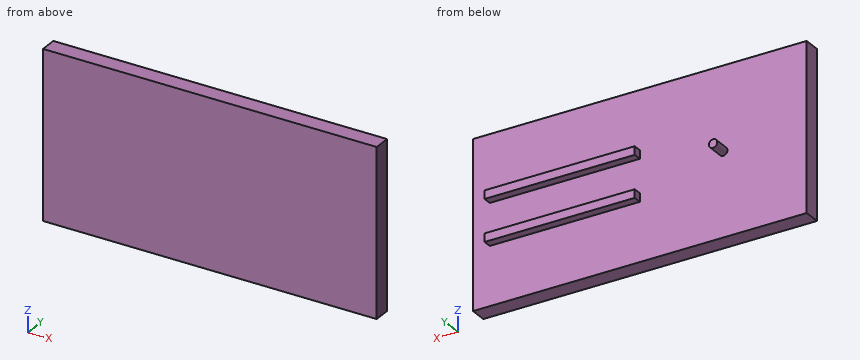
```python
from build123d import *

# Parameters (mm, degrees)
SKETCH1_W           = 200
SKETCH1_H           = 100
BOSS_EXTRUDE1_DEPTH = 10
SKETCH2_W           = 90
SKETCH2_H           = 5
BOSS_EXTRUDE2_DEPTH = 5
SKETCH2_3_R         = 2.5
BOSS_EXTRUDE3_DEPTH = 10


with BuildPart() as part:
    # Sketch1 → Boss-Extrude1 (new body)
    with BuildSketch(Plane(origin=(0, 0, 0), x_dir=(1, 0, 0), z_dir=(0, 1, 0))):
        Rectangle(SKETCH1_W, SKETCH1_H)
    extrude(amount=BOSS_EXTRUDE1_DEPTH)

    # Sketch2 → Boss-Extrude2 (add)
    with BuildSketch(Plane(origin=(0, 10, 0), x_dir=(1, 0, 0), z_dir=(0, 1, 0))):
        with Locations((45, 12.5)):
            Rectangle(SKETCH2_W, SKETCH2_H)
        with Locations((45, -12.5)):
            Rectangle(SKETCH2_W, SKETCH2_H)
    extrude(amount=BOSS_EXTRUDE2_DEPTH)

    # Sketch2_3 → Boss-Extrude3 (add)
    with BuildSketch(Plane(origin=(0, 10, 0), x_dir=(1, 0, 0), z_dir=(0, 1, 0))):
        with Locations(Location((-50, 0, 0), (0, 0, 90))):
            Circle(SKETCH2_3_R)
    extrude(amount=BOSS_EXTRUDE3_DEPTH)


solid = part.part
```
Build history of the part. All positions in model axes, mm. Round coordinates to 2 decimals unless told otherwise and drop trailing zeros. Order: outer loops, then holes, each group sorted by start corner. A loop starts at its lowest first (then second) coordinate and runs counter-clockwise, first axis right, second up. Notation, with made-up numbers: (21, 35.25) - (31, 35.25) arc R34 ccw to (31, 72.25) - close; hole circle Ø8 at (65.25, 1.5). An arc over 180 degrees is marked (long way). Use a Markdown table: item, result.
1) Flat gauge pins, fed straight in: pin 1 Ø1.5 at (x, y) = (36, 12) entering from -Z; pin 2 Ø10 at (x, z) = (-68, 10) entering from +Y; pin 3 Ø1.5 at (x, z) = (63.5, -12) entering from +Y. Where does each tip first touch, or does it go through?
Recorded:
| item | result |
|---|---|
| pin 1 | stops at z = -15 |
| pin 2 | stops at y = 10 |
| pin 3 | stops at y = 15 |
2) Saw through at A-A on y = 12.25. Write the cut outline in (x, z), and give its area (3 significant figures).
Recorded:
| item | result |
|---|---|
| outline | circle Ø5 at (-50, 0); (0, -15) - (90, -15) - (90, -10) - (0, -10) - close; (0, 10) - (90, 10) - (90, 15) - (0, 15) - close |
| area | 920 mm² |
3) Wall check: L1, parallel to Z at x = 84, y = 12.5; L2, parallel to Y at x = 53, z = -4; L3, parallel to X at y = 17.25, z = -1. Give the ranges that are in metal, low to high.
Recorded:
| item | result |
|---|---|
| L1 | z = -15 to -10, 10 to 15 |
| L2 | y = 0 to 10 |
| L3 | x = -52.29 to -47.71 |
4) Saw through at B-B on z = 0. Write the cut outline in (x, y), and give its area (3 significant figures).
Recorded:
| item | result |
|---|---|
| outline | (-100, 0) - (100, 0) - (100, 10) - (-47.5, 10) - (-47.5, 20) - (-52.5, 20) - (-52.5, 10) - (-100, 10) - close |
| area | 2,050 mm² |
5) Saw through at D-D on x = -41. Write the cut outline in (y, z).
Recorded:
| item | result |
|---|---|
| outline | (0, -50) - (10, -50) - (10, 50) - (0, 50) - close |
6) Saw through at C-C on x = 75. Write the cut outline in (y, z).
Recorded:
| item | result |
|---|---|
| outline | (0, -50) - (10, -50) - (10, -15) - (15, -15) - (15, -10) - (10, -10) - (10, 10) - (15, 10) - (15, 15) - (10, 15) - (10, 50) - (0, 50) - close |
